Can you work these out from the model? Positions are in its coordinate system, mm. Face numbers are marked on the shaded views. Give positions to 0.01 mm unless a question says otherwise; leave off trailing zeros. Order: outer loops, then holes, each group sorted by start corner. A loop starts at its lowest first (then second) coordinate and runs counter-clockwise, first axis right, second up. Notation, with made-up numbers: (25.25, 70) - (61.25, 70) arc R16 cw to (61.25, 90) - close; hole circle Ø6 at (83, 5.25). An arc over 180 degrees is marked (long way). Answer as CSV lines item,"result".
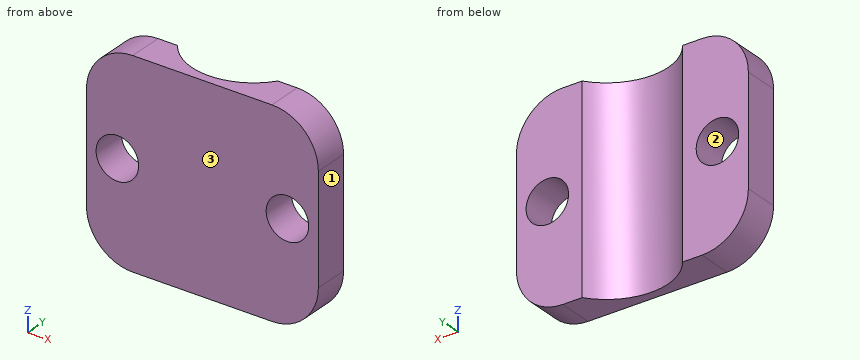
```python
from build123d import *

# Parameters (mm, degrees)
SKETCH1_W                      = 30
SKETCH1_H                      = 26
BOSS_EXTRUDE1_DEPTH            = 4.5
CUT_EXTRUDE1_DEPTH             = 40.953097502
F_5_5_5_5_DIAMETER_HOLE1_D     = 5.5
F_5_5_5_5_DIAMETER_HOLE1_DEPTH = 10
F_5_5_5_5_DIAMETER_HOLE1_TIP   = 1.652366702
FILLET2_R                      = 6


with BuildPart() as part:
    # Sketch1 → Boss-Extrude1 (new body)
    with BuildSketch(Plane(origin=(0, 0, 0), x_dir=(1, 0, 0), z_dir=(0, 1, 0))):
        with Locations((15, 13)):
            Rectangle(SKETCH1_W, SKETCH1_H)
    extrude(amount=BOSS_EXTRUDE1_DEPTH)

    # Sketch2 → Cut-Extrude1 (cut, through all)
    with BuildSketch(Plane.XY):
        with BuildLine():
            Line((8.5, 4.5), (21.5, 4.5))
            ThreePointArc((21.5, 4.5), (15, 1.163689527), (8.5, 4.5))
        make_face()
    extrude(amount=-CUT_EXTRUDE1_DEPTH, mode=Mode.SUBTRACT)

    # Ø5.5 (5.5) Diameter Hole1
    with Locations(Plane(origin=(0, 4.5, 0), x_dir=(-1, 0, 0), z_dir=(0, 1, 0))):
        with Locations((-4, -13), (-26, -13)):
            Hole(F_5_5_5_5_DIAMETER_HOLE1_D / 2, depth=F_5_5_5_5_DIAMETER_HOLE1_DEPTH)
            with Locations((0, 0, -(F_5_5_5_5_DIAMETER_HOLE1_DEPTH + F_5_5_5_5_DIAMETER_HOLE1_TIP / 2))):  # 118° drill point
                Cone(0, F_5_5_5_5_DIAMETER_HOLE1_D / 2, F_5_5_5_5_DIAMETER_HOLE1_TIP, mode=Mode.SUBTRACT)

    # Fillet2
    fillet2_edges = [part.edges().sort_by_distance(p)[0] for p in [
        (0, 2.25, 0),
        (0, 2.25, -26),
        (30, 2.25, -26),
        (30, 2.25, 0),
    ]]
    fillet(fillet2_edges, radius=FILLET2_R)


solid = part.part
```
1) If we mould it in two halves opening along X, with no side actions, what happens to the marked faces 1, 2 and 3? For each: +X half, -X half, draft (parallel to the pull), parting line (faces both ways), or undercut.
Answer block:
face 1,"+X half"
face 2,"undercut"
face 3,"draft"
2) I want a section at C-C on x = 4. Write out the boundary of the cut face in (y, z).
Answer block:
outline,"(0, -25.66) - (4.5, -25.66) - (4.5, -15.75) - (0, -15.75) - close; (0, -10.25) - (4.5, -10.25) - (4.5, -0.34) - (0, -0.34) - close"
3) I'm going to push a flat-ended pin straight in: P1, Ø1, axis at x = 16, y = 3, coming from the -Z side. Where does the tip first touch, or does it pass through?
Answer block:
P1,"through"
4) I want a section at A-A on y = 3.2. Write out the boundary of the cut face in (x, z), plus the area to 3 significant figures.
Answer block:
outline,"(0, -20) arc R6 ccw to (6, -26) - (9.67, -26) - (9.67, 0) - (6, 0) arc R6 ccw to (0, -6) - close; (20.33, -26) - (24, -26) arc R6 ccw to (30, -20) - (30, -6) arc R6 ccw to (24, 0) - (20.33, 0) - close; hole circle Ø5.5 at (4, -13); hole circle Ø5.5 at (26, -13)"
area,"424 mm2"
5) I want a section at D-D on z = -6.75. Write out the boundary of the cut face in (x, y).
Answer block:
outline,"(0, 0) - (30, 0) - (30, 4.5) - (21.5, 4.5) arc R8 cw to (8.5, 4.5) - (0, 4.5) - close"
6) I need wall thicknesses on line 1 along X through (y, z) = (2.9, -11); line 2 along X through (y, z) = (3.85, -15.25); line 3 along Z through (x, y) = (26, 1.8). Which ranges of each line are inside material? Lowest first, please. Write a range as [from, to].
Answer block:
line 1,"[0, 2.11], [5.89, 10.02], [19.98, 24.11], [27.89, 30]"
line 2,"[0, 2.42], [5.58, 9.02], [20.98, 24.42], [27.58, 30]"
line 3,"[-25.66, -15.75], [-10.25, -0.34]"
7) I want a section at B-B on z = -13. Write out the boundary of the cut face in (x, y).
Answer block:
outline,"(0, 0) - (1.25, 0) - (1.25, 4.5) - (0, 4.5) - close; (6.75, 0) - (23.25, 0) - (23.25, 4.5) - (21.5, 4.5) arc R8 cw to (8.5, 4.5) - (6.75, 4.5) - close; (28.75, 0) - (30, 0) - (30, 4.5) - (28.75, 4.5) - close"
